Work out the finished part from the listing and answer in its coordinate system (mm). A direction names the side the tool comes from. Give positions to 0.01 mm unless a question says otherwise; leave off trailing zeros. Write each loop counter-clockwise with the first axis right and the second up, starting at its lowest first coordinate (ties: lowest second). Pieces come first, ordered by that corner, then holes. Notation, with made-up numbers: (-5, -13) -> (27, -13) arc R16 cw to (27, 0) -> close; hole circle Ø10 at (29, 44.5). An arc over 180 degrees is marked (long way). Write item = value, one per line. Start each with the question number.
Autodesk Inventor part; units mm, degrees
ref_plane "YZ Plane" through (0, 0, 0) normal (1, 0, 0) x (0, 1, 0)
ref_plane "XZ Plane" through (0, 0, 0) normal (0, 1, 0) x (-1, 0, 0)
ref_plane "XY Plane" through (0, 0, 0) normal (0, 0, 1) x (1, 0, 0)
sketch "Sketch1" plane through (0, 0, 0) normal (0, 0, 1) x (1, 0, 0)
  line L0 (0, 0) -> (100, 0)
  line L1 (100, 0) -> (100, 20)
  line L2 (0, 0) -> (0, 100)
  line L3 (0, 100) -> (20, 100)
  line L4 (20, 100) -> (20, 20)
  line L5 (20, 20) -> (100, 20)
  dimension "d0" = 100
  dimension "d1" = 20
  dimension "d2" = 100
  dimension "d3" = 20
extrude "Extrusion1" add sketch "Sketch1" along normal mid plane 30
properties part number "CE-10.1.2" material "Stainless Steel"
(1) A cutting plane is placed at B-B, the plane x = 77. Write down the section's boundary in (y, z).
(2) For faces 1 (the flat face through (59, 20, 0)), 2 (the flat face through (10, 100, 0)), determine the directions among +Z, -Z, +X, -X, +Y, -Y from which every point of the face is accessible in a straight line to the end or side of a thin tool.
(3) Find the intervals of material crossed by line 1 along Y through (x, z) = (68.5, 2.25), in increasing order.
(4) A cutting plane is placed at A-A, the plane z = -4.5. Write down the section's boundary in (x, y).
(5) Each of these flat-tipped pins is pushed along its axis until it touches: pin 1 (12 mm diameter, centred on y = 85.5, z = 11, fed in from +X); pin 2 (12 mm diameter, centred on x = 75, z = -7, fed in from +Y); pin 3 (1.5 mm diameter, centred on x = 54, z = -6.5, fed in from -Y); pin 4 (2 mm diameter, centred on x = 21.5, y = 52, fed in from -Z). Where does it stop, or does it pass through?
Results list:
q1.outline = (0, -15) -> (20, -15) -> (20, 15) -> (0, 15) -> close
q2.face_1 = +Z, -Z, +X, +Y
q2.face_2 = +Z, -Z, +X, -X, +Y
q3.line_1 = 0 to 20
q4.outline = (0, 0) -> (100, 0) -> (100, 20) -> (20, 20) -> (20, 100) -> (0, 100) -> close
q5.pin_1 = 20
q5.pin_2 = 20
q5.pin_3 = 0
q5.pin_4 = through
